Design review of the part built by this model. Coordinates are the model's own, in mm. Face numbers are marked on the shaded views. A direction names the side the tool comes from. Give positions to 0.01 mm unless a question says otherwise; leave off trailing zeros. Write each loop counter-clockwise with the first axis right and the second up, starting at its lowest first coordinate (ties: lowest second). Pieces come first, ordered by that corner, then holes.
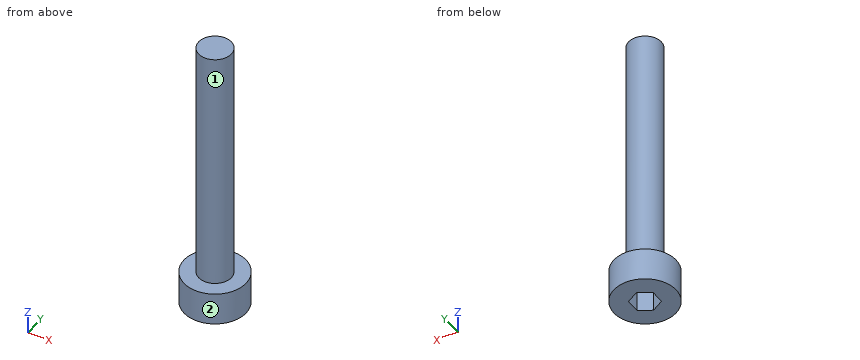
Autodesk Inventor part; units mm, degrees
ref_plane "YZ Plane" through (0, 0, 0) normal (1, 0, 0) x (0, 1, 0)
ref_plane "XZ Plane" through (0, 0, 0) normal (0, 1, 0) x (-1, 0, 0)
ref_plane "XY Plane" through (0, 0, 0) normal (0, 0, 1) x (1, 0, 0)
sketch "スケッチ1" plane through (0, 0, 0) normal (1, 0, 0) x (0, 1, 0)
  line L0 (0, 17) -> (0, 0)
  line L1 (0, 0) -> (1.9, 0)
  line L2 (1.9, 0) -> (1.9, 2)
  line L3 (1.9, 2) -> (1, 2)
  line L4 (1, 2) -> (1, 17)
  line L5 (1, 17) -> (0, 17)
  dimension "d1" = 1
  dimension "d2" = 2
  dimension "d3" = 1.9
  dimension "d10" = 15
revolve "回転1" add sketch "スケッチ1" angle 360 about axis through (0, 0, 17) along (0, 0, -1)
thread "ねじ1"
sketch "スケッチ2" plane through (0, 0, 0) normal (0, 0, -1) x (-1, 0, 0)
  line L0 (0, 0.866) -> (0.75, 0.433)
  line L1 (0.75, 0.433) -> (0.75, -0.433)
  line L2 (0.75, -0.433) -> (0, -0.866)
  line L3 (0, -0.866) -> (-0.75, -0.433)
  line L4 (-0.75, -0.433) -> (-0.75, 0.433)
  line L5 (-0.75, 0.433) -> (0, 0.866)
  line L6 (0, 1.9) -> (0, -1.9) construction
  point P0 (0, 0)
  point P1 (0, 0)
  dimension "d7" = 1.5
extrude "押し出し1" cut sketch "スケッチ2" against normal blind 1.4
properties part number "M2-15" material "ステンレス鋼 AISI 304"
(1) Clearance check with a flat-ended pin moving along its axis: P1, Ø1, axis at y = 0, z = 7, coming from the -X side. State where the tip first meets the part, or that it passes through.
Resolved:
P1: stops at x = -1
(2) Consider section C-C, the plane z = 5.5. Give the boundary of the cut face in (x, y).
Resolved:
outline: circle Ø2 at (0, 0)
(3) Tool access review of the marked faces 1 and 2: name each direction out of +Z, -Z, +X, -X, +Y, -Y from which nothing blocks a thin tool from reaching the whole face with its end or side.
Resolved:
face 1: +Z
face 2: +Z, -Z
(4) Consider section A-A, the plane y = 0. Give the boundary of the cut face in (x, z), then the cut area to 3 significant figures.
Resolved:
outline: (-1.9, 0) - (-0.75, 0) - (-0.75, 1.4) - (0.75, 1.4) - (0.75, 0) - (1.9, 0) - (1.9, 2) - (1, 2) - (1, 17) - (-1, 17) - (-1, 2) - (-1.9, 2) - close
area: 35.5 mm2
(5) To check wall thickness, follow L1, parallel to Y at x = 0.5, z = 14.75; L2, parallel to Z at x = 1.1, y = -0.7; L3, parallel to Z at x = -0.05, y = -0.5. State the ranges of each line that lie inside material, in increasing order.
Resolved:
L1: y = -0.87 to 0.87
L2: z = 0 to 2
L3: z = 1.4 to 17
(6) Consider section B-B, the plane x = 0.55. Give the boundary of the cut face in (y, z).
Resolved:
outline: (-1.82, 0) - (-0.55, 0) - (-0.55, 1.4) - (0.55, 1.4) - (0.55, 0) - (1.82, 0) - (1.82, 2) - (0.84, 2) - (0.84, 17) - (-0.84, 17) - (-0.84, 2) - (-1.82, 2) - close
(7) Consider section D-D, the plane x = 1.35. Give the boundary of the cut face in (y, z).
Resolved:
outline: (-1.34, 0) - (1.34, 0) - (1.34, 2) - (-1.34, 2) - close
